```python
from build123d import *

# Parameters (mm, degrees)
SKETCH1_W                       = 15.5
SKETCH1_H                       = 82.5
BOSS_EXTRUDE1_DEPTH             = 20
SKETCH2_R                       = 5.85
SKETCH2_R_2                     = 5.05
CUT_EXTRUDE1_DEPTH              = 10
FILLET1_R                       = 4
SKIZZE3_R                       = 5.1
SKIZZE3_R_2                     = 5.05
AUFSATZ_LINEAR_AUSTRAGEN1_DEPTH = 7.3
SCHNITT_LINEAR_AUSTRAGEN1_DEPTH = 9


with BuildPart() as part:
    # Sketch1 → Boss-Extrude1 (new body)
    with BuildSketch(Plane.XY):
        with Locations((-157.25, 123.75)):
            Rectangle(SKETCH1_W, SKETCH1_H)
    extrude(amount=BOSS_EXTRUDE1_DEPTH)

    # Sketch2 → Cut-Extrude1 (cut)
    with BuildSketch(Plane.XY.offset(20)):
        with BuildLine():
            ThreePointArc((-163.1, 123.75), (-157.25, 129.6), (-151.4, 123.75))
            Line((-151.4, 123.75), (-149.5, 123.75))
            Line((-149.5, 123.75), (-149.5, 165))
            Line((-149.5, 165), (-165, 165))
            Line((-165, 165), (-165, 123.75))
            Line((-165, 123.75), (-163.1, 123.75))
        make_face()
        with Locations((-157.25, 140.25)):
            Circle(SKETCH2_R, mode=Mode.SUBTRACT)
        with Locations((-157.25, 156.75)):
            Circle(SKETCH2_R, mode=Mode.SUBTRACT)
        with BuildLine():
            Line((-149.5, 123.75), (-151.4, 123.75))
            ThreePointArc((-151.4, 123.75), (-157.25, 117.9), (-163.1, 123.75))
            Line((-163.1, 123.75), (-165, 123.75))
            Line((-165, 123.75), (-165, 82.5))
            Line((-165, 82.5), (-149.5, 82.5))
            Line((-149.5, 82.5), (-149.5, 123.75))
        make_face()
        with Locations((-157.25, 90.75)):
            Circle(SKETCH2_R, mode=Mode.SUBTRACT)
        with Locations((-157.25, 107.25)):
            Circle(SKETCH2_R, mode=Mode.SUBTRACT)
        with Locations((-157.25, 90.75)):
            Circle(SKETCH2_R_2)
        with Locations((-157.25, 107.25)):
            Circle(SKETCH2_R_2)
        with BuildLine():
            ThreePointArc((-162.3, 123.75), (-157.25, 118.7), (-152.2, 123.75))
            Line((-152.2, 123.75), (-162.3, 123.75))
        make_face()
        with BuildLine():
            Line((-162.3, 123.75), (-152.2, 123.75))
            ThreePointArc((-152.2, 123.75), (-157.25, 128.8), (-162.3, 123.75))
        make_face()
        with Locations((-157.25, 140.25)):
            Circle(SKETCH2_R_2)
        with Locations((-157.25, 156.75)):
            Circle(SKETCH2_R_2)
    extrude(amount=-CUT_EXTRUDE1_DEPTH, mode=Mode.SUBTRACT)

    # Fillet1
    fillet1_edges = [part.edges().sort_by_distance(p)[0] for p in [
        (-165, 165, 5),
        (-149.5, 165, 5),
        (-149.5, 82.5, 5),
        (-165, 82.5, 5),
    ]]
    fillet(fillet1_edges, radius=FILLET1_R)

    # Skizze3 → Aufsatz-Linear austragen1 (add)
    with BuildSketch(Plane.XY.offset(10)):
        with Locations((-157.25, 156.75)):
            Circle(SKIZZE3_R)
        with Locations((-157.25, 140.25)):
            Circle(SKIZZE3_R)
        with Locations((-157.25, 123.75)):
            Circle(SKIZZE3_R_2)
        with Locations((-157.25, 107.25)):
            Circle(SKIZZE3_R_2)
        with Locations((-157.25, 90.75)):
            Circle(SKIZZE3_R)
    extrude(amount=AUFSATZ_LINEAR_AUSTRAGEN1_DEPTH)

    # Skizze4 → Schnitt-Linear austragen1 (cut)
    with BuildSketch(Plane(origin=(0, 0, 0), x_dir=(-1, 0, 0), z_dir=(0, 0, -1))):
        with BuildLine():
            Line((161, 163), (153.5, 163))
            ThreePointArc((153.5, 163), (152.085786438, 162.414213562), (151.5, 161))
            Line((151.5, 161), (151.5, 86.5))
            ThreePointArc((151.5, 86.5), (152.085786438, 85.085786438), (153.5, 84.5))
            Line((153.5, 84.5), (161, 84.5))
            ThreePointArc((161, 84.5), (162.414213562, 85.085786438), (163, 86.5))
            Line((163, 86.5), (163, 161))
            ThreePointArc((163, 161), (162.414213562, 162.414213562), (161, 163))
        make_face()
    extrude(amount=-SCHNITT_LINEAR_AUSTRAGEN1_DEPTH, mode=Mode.SUBTRACT)


solid = part.part
```
Input: part model. Units: mm. Frame: model coordinates. A direction names the side the tool comes from. Give positions to 0.01 mm unless a question says otherwise; leave off trailing zeros. Order: outer loops, then holes, each group sorted by start corner. A loop starts at its lowest first (then second) coordinate and runs counter-clockwise, first axis right, second up. Notation, with made-up numbers: (54, -8) - (62, -8) arc R14 cw to (62, 17) - close; hole circle Ø11 at (29.25, 66). An arc over 180 degrees is marked (long way). Use a Markdown table: item, result.
(1) Pin query (flat end, axial travel): pin 1 (3 mm diameter, centred on x = -159.5, y = 131.5, fed in from +Z); pin 2 (4 mm diameter, centred on x = -153, z = 16.5, fed in from -Y); pin 3 (8 mm diameter, centred on x = -157.25, y = 140.25, fed in from -Z). Return the tip coordinate at first contact, or that it passes through.
Computed values:
| item | result |
|---|---|
| pin 1 | stops at z = 10 |
| pin 2 | stops at y = 85.35 |
| pin 3 | stops at z = 9 |
(2) Draft query along Y for faces 1 (the cylindrical face through (-151.846, 138.009, 15.07)), 2 (the flat face through (-162, 154, 20)), 3 (the cylindrical face through (-150.703, 163.859, 5.07)). Return one class per face: released by +Y, released by -Y, zero draft, split by the parting line, or undercut.
Computed values:
| item | result |
|---|---|
| face 1 | undercut |
| face 2 | zero draft |
| face 3 | released by +Y |
(3) Section query D-D (y = 110). Output: boundary loops of the cut face in (x, z).
Computed values:
| item | result |
|---|---|
| outline | (-165, 0) - (-163, 0) - (-163, 9) - (-151.5, 9) - (-151.5, 0) - (-149.5, 0) - (-149.5, 10) - (-152.09, 10) - (-152.09, 20) - (-153.01, 20) - (-153.01, 17.3) - (-161.49, 17.3) - (-161.49, 20) - (-162.41, 20) - (-162.41, 10) - (-165, 10) - close |
(4) Access query for faces 4 (the flat face through (-162, 138, 20)), 5 (the flat face through (-157, 124, 9)), 6 (the cylindrical face through (-152.433, 92.267, 18.669)). Directions: +Z, -Z, +X, -X, +Y, -Y. A direction counts if a zero-diameter tool reaches every point of the face in a straight line with its end or side. Return the directions, or none.
Computed values:
| item | result |
|---|---|
| face 4 | +Z, +X, -X, +Y, -Y |
| face 5 | -Z |
| face 6 | +Z |
(5) Section query A-A (y = 131). Output: boundary loops of the cut face in (x, z), then the cut area to 3 significant figures.
Computed values:
| item | result |
|---|---|
| outline | (-165, 0) - (-163, 0) - (-163, 9) - (-151.5, 9) - (-151.5, 0) - (-149.5, 0) - (-149.5, 10) - (-165, 10) - close |
| area | 51.5 mm2 |
(6) Section query C-C (y = 156.75). Output: boundary loops of the cut face in (x, z), then the cut area to 3 significant figures.
Computed values:
| item | result |
|---|---|
| outline | (-165, 0) - (-163, 0) - (-163, 9) - (-151.5, 9) - (-151.5, 0) - (-149.5, 0) - (-149.5, 10) - (-151.4, 10) - (-151.4, 20) - (-152.2, 20) - (-152.2, 17.3) - (-162.3, 17.3) - (-162.3, 20) - (-163.1, 20) - (-163.1, 10) - (-165, 10) - close |
| area | 141 mm2 |
(7) Line query: line 1 (Y direction, x = -157, z = 13); line 2 (X direction, y = 130, z = 5.25); line 3 (Y direction, x = -160.5, z = 8.5). Output: solid intervals per line, ascending. Write a range as from..to.
Computed values:
| item | result |
|---|---|
| line 1 | y = 84.91..96.59, 101.41..113.09, 117.91..129.59, 134.41..146.09, 150.91..162.59 |
| line 2 | x = -165..-163, -151.5..-149.5 |
| line 3 | y = 82.5..84.5, 163..165 |
(8) Section query B-B (z = 16). Output: boundary loops of the cut face in (x, y).
Computed values:
| item | result |
|---|---|
| outline | circle Ø11.7 at (-157.25, 90.75); circle Ø11.7 at (-157.25, 107.25); circle Ø11.7 at (-157.25, 123.75); circle Ø11.7 at (-157.25, 140.25); circle Ø11.7 at (-157.25, 156.75) |
